Drawing for the job (mm, zero at the part's lowest x, y, z). A direction names the side the tool comes from. Give positions to 0.01 mm unless a question says otherwise; leave off trailing zeros. Write each loop counter-clockwise with the first axis right and the second up, starting at its lowest first coordinate (ties: lowest second). Pieces come first, ordered by that corner, then holes. Notation, with made-up numbers: M -37,-26 L 17,-26 A33 ccw 17,6 Z; hole C 12,47.5 d3. An arc over 180 degrees is marked long. Use a Markdown table: item, result. Add a question column.
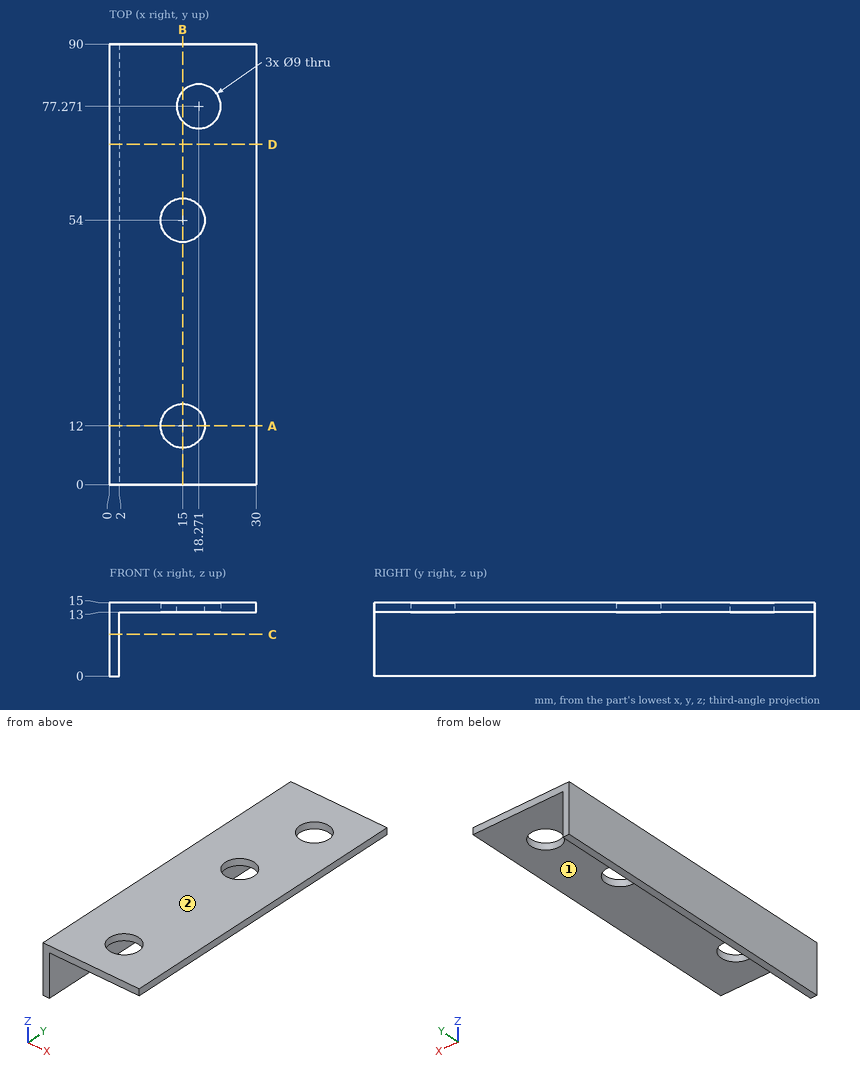
1. Cut at D-D (y = 69.5). Write the cut outline in (x, z).
2. Flat gauge pins, fed straight in: pin 1 (14.5 mm diameter, centred on x = 15, y = 54, fed in from -Z); pin 2 (8 mm diameter, centred on x = 15, y = 12, fed in from +Z); pin 3 (2 mm diameter, centred on y = 34, z = 5.5, fed in from +X); pin 4 (1.5 mm diameter, centred on y = 14, z = 8.5, fed in from -X). Where does each tip first touch, or does it go through?
3. Cut at B-B (x = 15). Write the cut outline in (y, z), then the cut area to 3 significant figures.
4. Cut at C-C (z = 8.5). Write the cut outline in (x, y), then the cut area to 3 significant figures.
5. Drill centre lines: probe 1 along X at (y, z) = (12, 14.55); probe 2 along Z at (x, y) = (7, 65.5); probe 3 along Y at (x, z) = (15, 13.65). Where is each one in solid material? Low to high. Write a range as [from, to].
6. Cut at A-A (y = 12). Write the cut outline in (x, z).
7. Tool access for the marked faces 1 and 2: list every direction of +Z, -Z, +X, -X, +Y, -Y with a clear straight run to the whole face (end or side of a thin tool).
A:
| question | item | result |
|---|---|---|
| 1 | outline | M 0,0 L 2,0 L 2,13 L 30,13 L 30,15 L 0,15 Z |
| 2 | pin 1 | stops at z = 13 |
| 2 | pin 2 | passes through |
| 2 | pin 3 | stops at x = 2 |
| 2 | pin 4 | stops at x = 0 |
| 3 | outline | M 0,13 L 7.5,13 L 7.5,15 L 0,15 Z; M 16.5,13 L 49.5,13 L 49.5,15 L 16.5,15 Z; M 58.5,13 L 74.18,13 L 74.18,15 L 58.5,15 Z; M 80.36,13 L 90,13 L 90,15 L 80.36,15 Z |
| 3 | area | 132 mm² |
| 4 | outline | M 0,0 L 2,0 L 2,90 L 0,90 Z |
| 4 | area | 180 mm² |
| 5 | probe 1 | x = [0, 10.5], [19.5, 30] |
| 5 | probe 2 | z = [13, 15] |
| 5 | probe 3 | y = [0, 7.5], [16.5, 49.5], [58.5, 74.18], [80.36, 90] |
| 6 | outline | M 0,0 L 2,0 L 2,13 L 10.5,13 L 10.5,15 L 0,15 Z; M 19.5,13 L 30,13 L 30,15 L 19.5,15 Z |
| 7 | face 1 | -Z, +X, +Y, -Y |
| 7 | face 2 | +Z, +X, -X, +Y, -Y |
